Input: dimensioned drawing with shaded views. Units: mm. Origin: part minimum x, y, z. A direction names the side the tool comes from. Round coordinates to 2 decimals unless told otherwise and drop trailing zeros. Order: outer loops, then holes, each group sorted by start corner. A loop starts at its lowest first (then second) coordinate and runs counter-clockwise, first axis right, second up. Notation, with made-up numbers: (-20.5, 89.25) -> (-12.5, 89.25) arc R24 ccw to (-12.5, 101.25) -> close; hole circle Ø1 at (-7, 5.5). An arc over 180 degrees is marked (long way). Use a Markdown table: item, result. Add a question column.
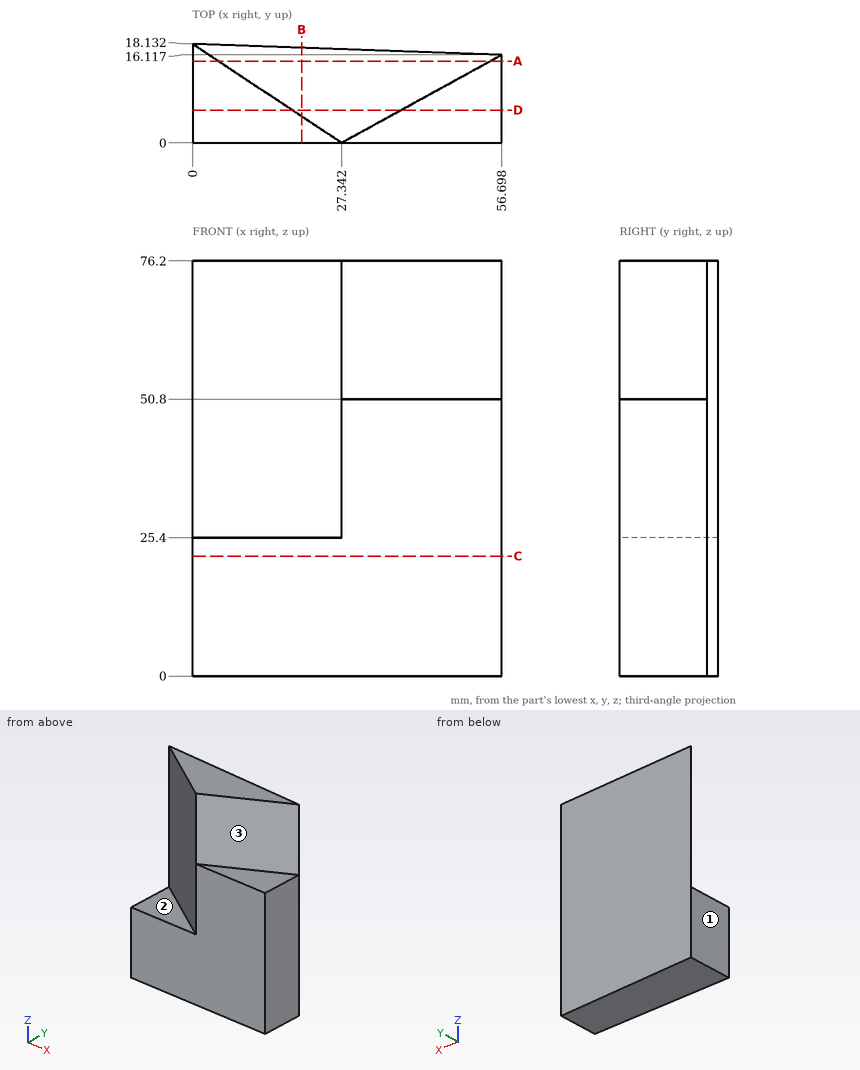
1) Reachability of the marked faces 1, 2 and 3 from +Z, -Z, +X, -X, +Y, -Y: full face, straight path, thin tool, end or side. Return the list, or none.
2) First-contact query: pin 1 Ø5 at (x, y) = (49, 9) entering from +Z; pin 2 Ø1 at (x, z) = (17, 61) entering from -Y; pin 3 Ø8 at (x, z) = (17, 23) entering from +Y. Flat tips, straight axial feed; report the tip coordinate or a pass-through.
3) Section A-A on y = 15. Output: boundary loops of the cut face in (x, z), then the cut area to 3 significant figures.
4) Section C-C on z = 22. Output: boundary loops of the cut face in (x, y).
5) Section D-D on y = 6. Output: boundary loops of the cut face in (x, z).
6) Section B-B on x = 20. Output: boundary loops of the cut face in (y, z).
7) Line query: probe 1 along Z at (x, y) = (5.5, 3.5); probe 2 along Z at (x, y) = (49, 1.25); probe 3 along Y at (x, z) = (46, 20.5). Output: solid intervals per line, ascending. Write a range as from..to.
Conclusion:
| question | item | result |
|---|---|---|
| 1 | face 1 | +Z, -Z, -X, +Y, -Y |
| 1 | face 2 | +Z, -X, -Y |
| 1 | face 3 | +Z, +X, -Y |
| 2 | pin 1 | stops at z = 50.8 |
| 2 | pin 2 | stops at y = 6.53 |
| 2 | pin 3 | stops at y = 17.67 |
| 3 | outline | (0, 0) -> (56.7, 0) -> (56.7, 50.8) -> (54.66, 50.8) -> (54.66, 76.2) -> (4.72, 76.2) -> (4.72, 25.4) -> (0, 25.4) -> close |
| 3 | area | 4,030 mm^2 |
| 4 | outline | (0, 0) -> (56.7, 0) -> (56.7, 16.12) -> (0, 18.13) -> close |
| 5 | outline | (0, 0) -> (56.7, 0) -> (56.7, 50.8) -> (38.27, 50.8) -> (38.27, 76.2) -> (18.29, 76.2) -> (18.29, 25.4) -> (0, 25.4) -> close |
| 6 | outline | (0, 0) -> (17.42, 0) -> (17.42, 76.2) -> (4.87, 76.2) -> (4.87, 25.4) -> (0, 25.4) -> close |
| 7 | probe 1 | z = 0..25.4 |
| 7 | probe 2 | z = 0..50.8 |
| 7 | probe 3 | y = 0..16.5 |
